Build history of the part. All positions in model axes, mm. Face numbers are marked on the shaded views. A direction names the side the tool comes from. Give positions to 0.01 mm unless a question says otherwise; leave off trailing zeros. Write each loop counter-clockwise with the first axis right and the second up, starting at its lowest first coordinate (ties: lowest second). Pieces come first, ordered by that corner, then holes. Notation, with made-up numbers: (-2, 8) -> (56, 8) arc R8 cw to (56, 20) -> close; hole circle Ø5 at (29, 83). An arc over 180 degrees is marked (long way). Write item = value, one per line. Start each with the question number.
Q1. Saw through at D-D, the plane z = 7.75. List the corners of the cut face in (x, y), then the cut area to 3 significant figures.
Q2. Tool access for the marked faces 1 and 2: list every direction of +Z, -Z, +X, -X, +Y, -Y with a clear straight run to the whole face (end or side of a thin tool).
Q3. Wall check: line 1 (Z direction, x = 1.75, y = 4); line 2 (Z direction, x = 3, y = 2.25); line 3 (Y direction, x = -1.75, z = 6.5). Give the ranges that are in metal, low to high.
Q4. Saw through at C-C, the plane z = 2.75. List the corners of the cut face in (x, y).
Q5. Drop flat-ended pins along their axis: P1, Ø1, axis at x = -5, y = -5, coming from the +Z side; P2, Ø2, axis at y = 1, z = 6, coming from the -X side; P3, Ø8.5, axis at x = -1, y = -4, coming from the +Z side; P4, Ø5, axis at y = 6, z = 6, coming from the +X side. Give the stop position or say it passes through.
Q6. Saw through at A-A, the plane y = 0. List the corners of the cut face in (x, z), then the cut area to 3 significant figures.
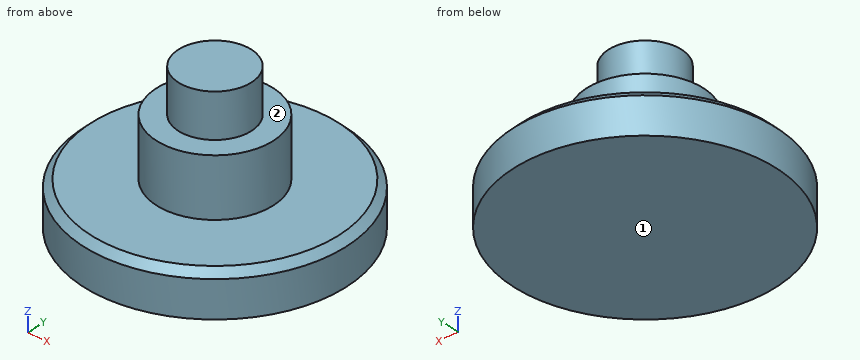
from build123d import *

# Parameters (mm, degrees)
F0_R     = 9
F1_DEPTH = 3
F2_SIZE  = 0.5
F3_R     = 4
F4_DEPTH = 4
F5_R     = 2.5
F6_DEPTH = 3


with BuildPart() as f1:
    # F0 (on Top) → F1 (new body)
    with BuildSketch(Plane.XY):
        Circle(F0_R)
    extrude(amount=F1_DEPTH)

    # F2
    f2_edges = [f1.edges().sort_by_distance(p)[0] for p in [
        (-9, 0, 3),
    ]]
    chamfer(f2_edges, length=F2_SIZE)

    # F3 (on face) → F4 (join)
    with BuildSketch(Plane.XY.offset(3)):
        Circle(F3_R)
    extrude(amount=F4_DEPTH)

    # F5 (on face) → F6 (join)
    with BuildSketch(Plane.XY.offset(7)):
        Circle(F5_R)
    extrude(amount=F6_DEPTH)


solid = f1.part
Report:
q1.outline = circle Ø5 at (0, 0)
q1.area = 19.6 mm2
q2.face_1 = -Z, +X, -X, +Y, -Y
q2.face_2 = +Z
q3.line_1 = 0 to 3
q3.line_2 = 0 to 7
q3.line_3 = -3.6 to 3.6
q4.outline = circle Ø17.5 at (0, 0)
q5.P1 = 3
q5.P2 = -4
q5.P3 = 10
q5.P4 = 1.94
q6.outline = (-9, 0) -> (9, 0) -> (9, 2.5) -> (8.5, 3) -> (4, 3) -> (4, 7) -> (2.5, 7) -> (2.5, 10) -> (-2.5, 10) -> (-2.5, 7) -> (-4, 7) -> (-4, 3) -> (-8.5, 3) -> (-9, 2.5) -> close
q6.area = 101 mm2
